from build123d import *

# Parameters (mm, degrees)
SKETCH_1_R      = 5.1
SKETCH_1_R_2    = 2.1
EXTRUDE_1_DEPTH = 4
EXTRUDE_2_DEPTH = 11.5
SKETCH_3_R      = 2
EXTRUDE_3_DEPTH = 4


with BuildPart() as part:
    # 草圖1 → 填料-伸長1 (new body)
    # profile 1 of 5: a face of its own
    with BuildSketch(Plane.XY):
        with Locations((-14.5, 11.5)):
            Circle(SKETCH_1_R)
        with Locations((-14.5, 11.5)):
            Circle(SKETCH_1_R_2, mode=Mode.SUBTRACT)
    # profile 2 of 5: a face of its own
    with BuildSketch(Plane.XY):
        with BuildLine():
            add(Edge.make_bspline(
                [(-9.4, 11.5), (0, 0.5), (9.4, 11.5)],
                knots=[0, 0, 0, 1, 1, 1], degree=2))
            ThreePointArc((-9.4, 11.5), (-10.893755416, 7.893755416), (-14.5, 6.4))
            add(Edge.make_bspline(
                [(-14.5, 6.4), (-5.5, 0), (-14.5, -6.4)],
                knots=[0, 0, 0, 1, 1, 1], degree=2))
            ThreePointArc((-14.5, -6.4), (-10.893755416, -7.893755416), (-9.4, -11.5))
            add(Edge.make_bspline(
                [(-9.4, -11.5), (0, -0.5), (9.4, -11.5)],
                knots=[0, 0, 0, 1, 1, 1], degree=2))
            ThreePointArc((9.4, -11.5), (10.893755416, -7.893755416), (14.5, -6.4))
            add(Edge.make_bspline(
                [(14.5, 6.4), (5.5, 0), (14.5, -6.4)],
                knots=[0, 0, 0, 1, 1, 1], degree=2))
            ThreePointArc((14.5, 6.4), (10.893755416, 7.893755416), (9.4, 11.5))
        make_face()
    # profile 3 of 5: a face of its own
    with BuildSketch(Plane.XY):
        with Locations((14.5, 11.5)):
            Circle(SKETCH_1_R)
        with Locations((14.5, 11.5)):
            Circle(SKETCH_1_R_2, mode=Mode.SUBTRACT)
    # profile 4 of 5: a face of its own
    with BuildSketch(Plane.XY):
        with Locations((14.5, -11.5)):
            Circle(SKETCH_1_R)
        with Locations((14.5, -11.5)):
            Circle(SKETCH_1_R_2, mode=Mode.SUBTRACT)
    # profile 5 of 5: a face of its own
    with BuildSketch(Plane.XY):
        with Locations((-14.5, -11.5)):
            Circle(SKETCH_1_R)
        with Locations((-14.5, -11.5)):
            Circle(SKETCH_1_R_2, mode=Mode.SUBTRACT)
    extrude(amount=EXTRUDE_1_DEPTH)

    # 草圖2 → 填料-伸長2 (add)
    with BuildSketch(Plane.XY.offset(4)):
        with BuildLine():
            ThreePointArc((-14.5, 6.4), (-10.893755416, 7.893755416), (-9.4, 11.5))
            add(Edge.make_bspline(
                [(9.4, 11.5), (0, 0.5), (-9.4, 11.5)],
                knots=[0, 0, 0, 1, 1, 1], degree=2))
            ThreePointArc((9.4, 11.5), (10.893755425, 7.893755407), (14.500000025, 6.400000018))
            add(Edge.make_bspline(
                [(14.5, -6.4), (5.499999987, 9e-09), (14.500000025, 6.400000018)],
                knots=[0, 0, 0, 1, 1, 1], degree=2))
            ThreePointArc((14.5, -6.4), (10.893755423, -7.893755409), (9.399999984, -11.499999981))
            add(Edge.make_bspline(
                [(-9.4, -11.5), (-8e-09, -0.500000009), (9.399999984, -11.499999981)],
                knots=[0, 0, 0, 1, 1, 1], degree=2))
            ThreePointArc((-9.4, -11.5), (-10.893755425, -7.893755407), (-14.500000025, -6.400000018))
            add(Edge.make_bspline(
                [(-14.5, 6.4), (-5.499999987, -9e-09), (-14.500000025, -6.400000018)],
                knots=[0, 0, 0, 1, 1, 1], degree=2))
        make_face()
    extrude(amount=EXTRUDE_2_DEPTH)

    # 草圖3 → 填料-伸長3 (add)
    with BuildSketch(Plane.XY.offset(15.5)):
        with BuildLine():
            Line((-20.5, 16.5), (20.5, 16.5))
            ThreePointArc((20.5, 16.5), (21.914213562, 15.914213562), (22.5, 14.5))
            Line((22.5, 14.5), (22.5, -26.5))
            ThreePointArc((22.5, -26.5), (21.914213562, -27.914213562), (20.5, -28.5))
            Line((20.5, -28.5), (-20.5, -28.5))
            ThreePointArc((-20.5, -28.5), (-21.914213562, -27.914213562), (-22.5, -26.5))
            Line((-22.5, -26.5), (-22.5, 14.5))
            ThreePointArc((-22.5, 14.5), (-21.914213562, 15.914213562), (-20.5, 16.5))
        make_face()
        with Locations((-18.5, 12.5)):
            Circle(SKETCH_3_R, mode=Mode.SUBTRACT)
        with Locations((-18.5, -24.5)):
            Circle(SKETCH_3_R, mode=Mode.SUBTRACT)
        with Locations((18.5, -24.5)):
            Circle(SKETCH_3_R, mode=Mode.SUBTRACT)
        with Locations((18.5, 12.5)):
            Circle(SKETCH_3_R, mode=Mode.SUBTRACT)
    extrude(amount=-EXTRUDE_3_DEPTH)


solid = part.part
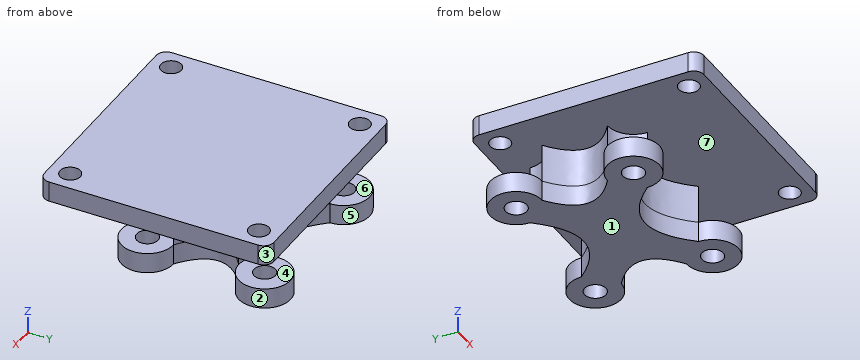
The listing builds one solid part. Answer for the finished solid, in the listing's coordinates (mm). Face numbers are marked on the shaded views. A direction names the side the tool comes from. Round coordinates to 2 decimals unless told otherwise and drop trailing zeros. Loops run counter-clockwise (first coordinate to the right, second up) from the corner with the lowest first, then second, coordinate; pieces in that order, holes last. Notation, with made-up numbers: M 38,-6 L 81,-6 A19 cw 81,19 Z; hole C -3,16 d10. An arc over 180 degrees is marked long. Write each question's results on one line, items separated by ' | '. Start each with the question number.
1) Each of these flat-tipped pins is pushed along its axis until it touches: pin 1 (3 mm diameter, centred on x = -17, z = 2.5, fed in from -Y); pin 2 (2 mm diameter, centred on x = 3, z = 13, fed in from +Y); pin 3 (5.5 mm diameter, centred on x = -14.5, y = 11.5, fed in from -Z); pin 4 (2.5 mm diameter, centred on x = 14.5, y = -11.5, fed in from -Z). Where does it stop, or does it pass through?
2) Find section B-B on z = 14.25. Write down the section's boundary in (x, y).
3) Find section A-A on y = -24.5. Write down the section's boundary in (x, z), plus the area to 3 significant figures.
4) Find section D-D on y = 12.5. Write down the section's boundary in (x, z).
5) Straight lines are drawn through the part: probe 1 along Y at (x, z) = (-14.5, 1.65); probe 2 along Y at (x, z) = (18.5, 12.85); probe 3 along Z at (x, y) = (-12, 10). For each, find the intervals that lie inside material, in ascending order.
6) Which of the six approach directions +Z, -Z, +X, -X, +Y, -Y give full straight-line access (tool end or side, diameter ignored) to the marked faces 4, 5, 6 and 7?
7) Determine the mould class of the marked faces 1, 2 and 3 for opening direction X: pulls with the +X half, pulls with the -X half, needs draft (parallel to the pull), parting line crosses it, or undercut.
8) Find section C-C on x = 18.5. Write down the section's boundary in (y, z).
Final values:
1) pin 1: y = -16.5 | pin 2: y = 16.5 | pin 3: z = 0 | pin 4: z = 11.5
2) outline: M -22.5,-26.5 A2 ccw -20.5,-28.5 L 20.5,-28.5 A2 ccw 22.5,-26.5 L 22.5,14.5 A2 ccw 20.5,16.5 L -20.5,16.5 A2 ccw -22.5,14.5 Z; hole C -18.5,-24.5 d4; hole C -18.5,12.5 d4; hole C 18.5,-24.5 d4; hole C 18.5,12.5 d4
3) outline: M -22.5,11.5 L -20.5,11.5 L -20.5,15.5 L -22.5,15.5 Z; M -16.5,11.5 L 16.5,11.5 L 16.5,15.5 L -16.5,15.5 Z; M 20.5,11.5 L 22.5,11.5 L 22.5,15.5 L 20.5,15.5 Z | area: 148 mm²
4) outline: M -22.5,11.5 L -20.5,11.5 L -20.5,15.5 L -22.5,15.5 Z; M -19.5,0 L -16.35,0 L -16.35,4 L -19.5,4 Z; M -16.5,11.5 L 16.5,11.5 L 16.5,15.5 L -16.5,15.5 Z; M -12.65,0 L -9.5,0 L -9.5,4 L -12.65,4 Z; M 9.5,0 L 12.65,0 L 12.65,4 L 9.5,4 Z; M 16.35,0 L 19.5,0 L 19.5,4 L 16.35,4 Z; M 20.5,11.5 L 22.5,11.5 L 22.5,15.5 L 20.5,15.5 Z
5) probe 1: -16.6 to -13.6, -9.4 to -6.4, 6.4 to 9.4, 13.6 to 16.6 | probe 2: -28.5 to -26.5, -22.5 to 10.5, 14.5 to 16.5 | probe 3: 0 to 4, 11.5 to 15.5
6) face 4: +X, +Y | face 5: -Z | face 6: -X, +Y | face 7: none
7) face 1: needs draft | face 2: undercut | face 3: pulls with the +X half
8) outline: M -28.5,11.5 L -26.5,11.5 L -26.5,15.5 L -28.5,15.5 Z; M -22.5,11.5 L 10.5,11.5 L 10.5,15.5 L -22.5,15.5 Z; M -14.66,0 L -8.34,0 L -8.34,4 L -14.66,4 Z; M 8.34,0 L 14.66,0 L 14.66,4 L 8.34,4 Z; M 14.5,11.5 L 16.5,11.5 L 16.5,15.5 L 14.5,15.5 Z
